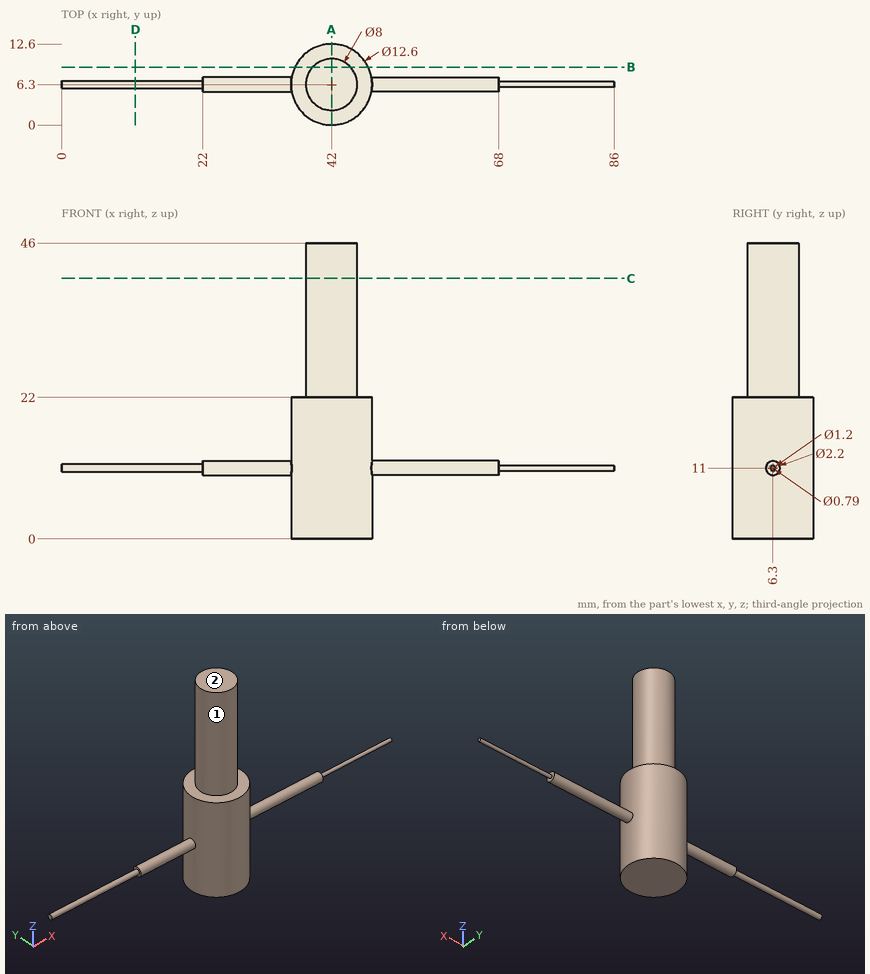
Geometry check sheet. Reference: drawing and pictorial views, mm from the part's lowest x, y, z. A direction names the side the tool comes from. Round coordinates to 2 decimals unless told otherwise and drop trailing zeros. Loops run counter-clockwise (first coordinate to the right, second up) from the corner with the lowest first, then second, coordinate; pieces in that order, holes last. Notation, with made-up numbers: (-20, 33) -> (2, 33) arc R22 cw to (2, 41) -> close; hole circle Ø10 at (26.25, -29.5). An arc over 180 degrees is marked (long way). Use a Markdown table: item, result.
(1) Go/stop test with flat-tipped pins: P1, Ø1, axis at x = 26, z = 14, coming from the +Y side; P2, Ø5, axis at y = 1.5, z = 8.5, coming from the +X side (1 decimal). Record where each tip stops, or that it passes through.
Calculated:
| item | result |
|---|---|
| P1 | through |
| P2 | x = 47.9 |
(2) Sectioned sample at D-D (x = 11.5). Enter the section's corners in (y, z), then the cut area to 3 significant figures.
Calculated:
| item | result |
|---|---|
| outline | circle Ø1.2 at (6.3, 11) |
| area | 1.13 mm² |
(3) Sectioned sample at C-C (z = 40.5). Enter the section's corners in (x, y), then the cut area to 3 significant figures.
Calculated:
| item | result |
|---|---|
| outline | circle Ø8 at (42, 6.3) |
| area | 50.3 mm² |
(4) Sectioned sample at A-A (x = 42). Enter the section's corners in (y, z).
Calculated:
| item | result |
|---|---|
| outline | (0, 0) -> (12.6, 0) -> (12.6, 22) -> (10.3, 22) -> (10.3, 46) -> (2.3, 46) -> (2.3, 22) -> (0, 22) -> close |
(5) Set-up check for the marked faces 1 and 2: record each of +Z, -Z, +X, -X, +Y, -Y from which the full face is reachable in a straight line by a thin tool's end or side.
Calculated:
| item | result |
|---|---|
| face 1 | +Z |
| face 2 | +Z, +X, -X, +Y, -Y |
(6) Sectioned sample at B-B (y = 9). Enter the section's corners in (x, z), then the cut area to 3 significant figures.
Calculated:
| item | result |
|---|---|
| outline | (36.31, 0) -> (47.69, 0) -> (47.69, 22) -> (44.95, 22) -> (44.95, 46) -> (39.05, 46) -> (39.05, 22) -> (36.31, 22) -> close |
| area | 392 mm² |
(7) Scan lines: probe 1 along Z at (x, y) = (45, 9.5); probe 2 along X at (y, z) = (5.25, 13); probe 3 along X at (y, z) = (6.25, 18.5). Record each from-to range of solid material in increasing order.
Calculated:
| item | result |
|---|---|
| probe 1 | 0 to 22 |
| probe 2 | 35.79 to 48.21 |
| probe 3 | 35.7 to 48.3 |
